from build123d import *

# Parameters (mm, degrees)
F0_W     = 17
F0_H     = 8
F1_DEPTH = 55
F2_R     = 1
F3_W     = 12.4
F3_H     = 5
F4_DEPTH = 14
F6_DEPTH = 25


with BuildPart() as f1:
    # F0 (on Front) → F1 (new body)
    with BuildSketch(Plane.XZ):
        Rectangle(F0_W, F0_H)
    extrude(amount=F1_DEPTH)

    # F2
    f2_edges = [f1.edges().sort_by_distance(p)[0] for p in [
        (-8.5, -27.5, 4),
        (-8.5, -27.5, -4),
        (8.5, -27.5, -4),
        (8.5, -27.5, 4),
    ]]
    fillet(f2_edges, radius=F2_R)

    # F3 (on face) → F4 (cut)
    with BuildSketch(Plane.XZ.offset(55)):
        Rectangle(F3_W, F3_H)
    extrude(amount=-F4_DEPTH, mode=Mode.SUBTRACT)

    # F5 (on face) → F6 (cut)
    with BuildSketch(Plane.XY.offset(4)):
        with BuildLine():
            ThreePointArc((5.091245, -9.798271), (3.965953, -5.706329), (0, -7.216787))
            ThreePointArc((0, -7.216787), (-4.103388, -5.665551), (-5.093883, -9.939079))
            Line((-5.093883, -9.939079), (0, -15.008175))
            Line((0, -15.008175), (5.091245, -9.798271))
        make_face()
    extrude(amount=-F6_DEPTH, mode=Mode.SUBTRACT)


solid = f1.part
Check sheet for the modelled part. Datum: model origin and axes. Units: mm. A direction names the side the tool comes from. Round coordinates to 2 decimals unless told otherwise and drop trailing zeros. Write each loop counter-clockwise with the first axis right and the second up, starting at its lowest first coordinate (ties: lowest second). Pieces come first, ordered by that corner, then holes. Notation, with made-up numbers: (79, -17.75) - (97, -17.75) arc R21 ccw to (97, -2.75) - close; hole circle Ø3 at (24.25, 85). An arc over 180 degrees is marked (long way). Return JSON: item names as keys, results as strings.
Q1. Cross-section at B-B (x = 0.5). Record the boundary of the cut face in (y, z), then the cut area to 3 significant figures.
Returned:
{"outline": "(-55, -4) - (-14.5, -4) - (-14.5, 4) - (-55, 4) - (-55, 2.5) - (-41, 2.5) - (-41, -2.5) - (-55, -2.5) - close; (-6.39, -4) - (0, -4) - (0, 4) - (-6.39, 4) - close", "area": "305 mm²"}
Q2. Depth check by flat-ended pin: P1, Ø4, axis at x = -2, z = 1, coming from the -Y side. Enter the tip coordinate at first touch or a pass-through.
Returned:
{"P1": "stops at y = -55"}
Q3. Cross-section at D-D (x = -2.5). Record the boundary of the cut face in (y, z).
Returned:
{"outline": "(-55, -4) - (-12.52, -4) - (-12.52, 4) - (-55, 4) - (-55, 2.5) - (-41, 2.5) - (-41, -2.5) - (-55, -2.5) - close; (-5.33, -4) - (0, -4) - (0, 4) - (-5.33, 4) - close"}
Q4. Access from +Z, -Z, +X, -X, +Y, -Y to the whole of each face (thin tool, end or side, straight path). Record for faces 1 (the flat face through (-2.58, -12.44, 0.06)), 2 (the flat face through (0, -27, -4)), 3 (the flat face through (0, -48, -2.5)).
Returned:
{"face 1": "+Z, -Z", "face 2": "-Z, +X, -X, +Y, -Y", "face 3": "-Y"}
Q5. Scan lines: L1, parallel to X at y = -44.5, z = 0.75; L2, parallel to Z at x = -1.75, y = -50; L3, parallel to Y at x = 0.5, z = 3.25. Record each from-to range of solid material in increasing order. Write a range as from..to.
Returned:
{"L1": "x = -8.5..-6.2, 6.2..8.5", "L2": "z = -4..-2.5, 2.5..4", "L3": "y = -55..-14.5, -6.39..0"}
Q6. Cross-section at C-C (z = -3.5). Record the boundary of the cut face in (x, y).
Returned:
{"outline": "(-8.37, -55) - (8.37, -55) - (8.37, 0) - (-8.37, 0) - close; hole (-5.09, -9.94) - (0, -15.01) - (5.09, -9.8) arc R2.87 ccw (long way) to (0, -7.22) arc R2.91 ccw (long way) to start"}
Q7. Draft check along Z on faces 4 (the cylindrical face through (8.199, -27.885, -3.715)), 5 (the flat face through (0, -55, 3)), 6 (the flat face through (0, -41, 0)). Enter one of: released by +Z, released by -Z, zero draft, split by the parting line, or undercut.
Returned:
{"face 4": "released by -Z", "face 5": "zero draft", "face 6": "undercut"}
Q8. Cross-section at A-A (y = -51). Record the boundary of the cut face in (x, z), then the cut area to 3 significant figures.
Returned:
{"outline": "(-8.5, -3) arc R1 ccw to (-7.5, -4) - (7.5, -4) arc R1 ccw to (8.5, -3) - (8.5, 3) arc R1 ccw to (7.5, 4) - (-7.5, 4) arc R1 ccw to (-8.5, 3) - close; hole (-6.2, -2.5) - (6.2, -2.5) - (6.2, 2.5) - (-6.2, 2.5) - close", "area": "73.1 mm²"}
